Part model, mm, in its own coordinate system. Round coordinates to 2 decimals unless told otherwise and drop trailing zeros. Order: outer loops, then holes, each group sorted by start corner. A loop starts at its lowest first (then second) coordinate and runs counter-clockwise, first axis right, second up. Notation, with made-up numbers: (75, -18.5) - (90, -18.5) arc R16 cw to (90, 10.5) - close; hole circle Ø1 at (-7.75, -21). An arc over 180 degrees is marked (long way). Return JSON: item names as keys, results as strings. Group by question number.
Item 1: Two-plate mould, pull along X, no slides. Class faces 1 (the face through (80, 7, 1)), 2 (the face through (-1, 15, -1)), 3 (the face through (-12.39, 10.76, 20.32)), 4 (the face through (64.581, 5.196, -28.794)): released by +X, released by -X, zero draft, split by the parting line, or undercut.
Item 2: Saw through at B-B on z = -25. List the corners of the cut face in (x, y).
Item 3: Saw through at D-D on z = 0. List the corners of the cut face in (x, y), and give its area (3 significant figures).
Item 4: Saw through at C-C on y = 3. State how many separate pieces and enclosed holes the cut face has, and give its area (3 significant figures).
Item 5: Saw through at A-A on x = 0. List the corners of the cut face in (y, z), and give its area (4 significant figures).
Item 6: Probe probe 1 along Z at (x, y) = (-67, 4.5); probe 2 along X at (y, z) = (5, -33.75); probe 3 along Z at (x, y) = (14.5, 8.25). List the from-to ranges inside material, lowest first.
Item 7: Drop flat-ended pins along their axis: pin 1 (11.5 mm diameter, centred on x = -13, z = -25, fed in from +Y); pin 2 (14.5 mm diameter, centred on x = 13, z = 25, fed in from +Y). Give the stop position or say it passes through.
```python
from build123d import *

# Parameters (mm, degrees)
DODANIE_WYCI_GNI_CIE1_DEPTH                        = 15
SZKIC2_R                                           = 4
WYTNIJ_WYCI_GNI_CIE1_DEPTH                         = 103.621878759
LUSTRO2_COPY_1_SKETCH_R                            = 4
LUSTRO2_COPY_1_DEPTH                               = 103.621878759
SFAZOWANIE1_SIZE                                   = 0.5
POG_BIENIE_STO_KOWE_POD_M8_WKR_T_Z_BEM_D           = 9
POG_BIENIE_STO_KOWE_POD_M8_WKR_T_Z_BEM_CSINK_D     = 17.92
POG_BIENIE_STO_KOWE_POD_M8_WKR_T_Z_BEM_CSINK_ANGLE = 90
SZKIC5_R                                           = 4
WYTNIJ_WYCI_GNI_CIE2_DEPTH                         = 103.621878759


with BuildPart() as part:
    # Szkic1 → Dodanie-wyciągnięcie1 (new body)
    with BuildSketch(Plane(origin=(0, 0, 0), x_dir=(1, 0, 0), z_dir=(0, 1, 0))):
        with BuildLine():
            Line((-70, -62.5), (70, -62.5))
            ThreePointArc((70, -62.5), (77.071067812, -59.571067812), (80, -52.5))
            Line((80, -52.5), (80, 52.5))
            ThreePointArc((80, 52.5), (77.071067812, 59.571067812), (70, 62.5))
            Line((70, 62.5), (-70, 62.5))
            ThreePointArc((-70, 62.5), (-77.071067812, 59.571067812), (-80, 52.5))
            Line((-80, 52.5), (-80, -52.5))
            ThreePointArc((-80, -52.5), (-77.071067812, -59.571067812), (-70, -62.5))
        make_face()
    extrude(amount=DODANIE_WYCI_GNI_CIE1_DEPTH)

    # Szkic2 → Wytnij-wyciągnięcie1 (cut, symmetric)
    with BuildSketch(Plane(origin=(0, 15, 0), x_dir=(1, 0, 0), z_dir=(0, 1, 0))):
        with Locations(Location((-67, -25, 0), (0, 0, 270))):
            Circle(SZKIC2_R)
        with Locations(Location((-13, -25, 0), (0, 0, 90))):
            Circle(SZKIC2_R)
    wytnij_wyci_gni_cie1 = extrude(amount=WYTNIJ_WYCI_GNI_CIE1_DEPTH, both=True, mode=Mode.SUBTRACT)

    # Lustro1: Wytnij-wyciągnięcie1 across plane
    add(wytnij_wyci_gni_cie1.mirror(Plane.XY), mode=Mode.SUBTRACT)

    # Lustro2: Wytnij-wyciągnięcie1 across plane
    add(wytnij_wyci_gni_cie1.mirror(Plane(origin=(0, 0, 0), x_dir=(0, 0, 1), z_dir=(1, 0, 0))), mode=Mode.SUBTRACT)

    # Lustro2 copy 1 sketch → Lustro2 copy 1 (cut, symmetric)
    with BuildSketch(Plane(origin=(0, 15, 0), x_dir=(-1, 0, 0), z_dir=(0, 1, 0))):
        with Locations(Location((-67, -25, 0), (0, 0, 270))):
            Circle(LUSTRO2_COPY_1_SKETCH_R)
        with Locations(Location((-13, -25, 0), (0, 0, 90))):
            Circle(LUSTRO2_COPY_1_SKETCH_R)
    extrude(amount=LUSTRO2_COPY_1_DEPTH, both=True, mode=Mode.SUBTRACT)

    # Sfazowanie1
    sfazowanie1_edges = [part.edges().sort_by_distance(p)[0] for p in [
        (-67, 0, 21),
        (-67, 15, 21),
        (-13, 0, 29),
        (-13, 15, 29),
        (-67, 15, -21),
        (-67, 0, -21),
        (-13, 15, -29),
        (-13, 0, -29),
        (67, 0, -21),
        (67, 15, -21),
        (13, 0, -29),
        (13, 15, -29),
        (67, 15, 21),
        (67, 0, 21),
        (13, 15, 29),
        (13, 0, 29),
    ]]
    chamfer(sfazowanie1_edges, length=SFAZOWANIE1_SIZE)

    # Pogłębienie stożkowe pod M8 Wkręt z łbem stożkowym płaskim1 (through all)
    with Locations(Plane(origin=(0, 15, 0), x_dir=(1, 0, 0), z_dir=(0, 1, 0))):
        with Locations((-67, 25), (-13, 25), (-13, -25), (13, -25), (13, 25), (67, 25), (67, -25), (-67, -25)):
            CounterSinkHole(POG_BIENIE_STO_KOWE_POD_M8_WKR_T_Z_BEM_D / 2, POG_BIENIE_STO_KOWE_POD_M8_WKR_T_Z_BEM_CSINK_D / 2, counter_sink_angle=POG_BIENIE_STO_KOWE_POD_M8_WKR_T_Z_BEM_CSINK_ANGLE)

    # Szkic5 → Wytnij-wyciągnięcie2 (cut, through all)
    with BuildSketch(Plane(origin=(0, 15, 0), x_dir=(1, 0, 0), z_dir=(0, 1, 0))):
        with Locations(Location((0, 33.75, 0), (0, 0, 270))):
            Circle(SZKIC5_R)
        with Locations(Location((33.75, 0, 0), (0, 0, 270))):
            Circle(SZKIC5_R)
        with Locations(Location((0, -33.75, 0), (0, 0, 270))):
            Circle(SZKIC5_R)
        with Locations(Location((-33.75, 0, 0), (0, 0, 270))):
            Circle(SZKIC5_R)
    extrude(amount=-WYTNIJ_WYCI_GNI_CIE2_DEPTH, mode=Mode.SUBTRACT)


solid = part.part
```
Filled in:
{
 "1": {"face 1": "released by +X", "face 2": "zero draft", "face 3": "undercut", "face 4": "undercut"},
 "2": {"outline": "(-80, 0) - (-71.5, 0) - (-71.5, 10.54) - (-75.96, 15) - (-80, 15) - close; (-62.5, 0) - (-17.5, 0) - (-17.5, 10.54) - (-21.96, 15) - (-58.04, 15) - (-62.5, 10.54) - close; (-8.5, 0) - (8.5, 0) - (8.5, 10.54) - (4.04, 15) - (-4.04, 15) - (-8.5, 10.54) - close; (17.5, 0) - (62.5, 0) - (62.5, 10.54) - (58.04, 15) - (21.96, 15) - (17.5, 10.54) - close; (71.5, 0) - (80, 0) - (80, 15) - (75.96, 15) - (71.5, 10.54) - close"},
 "3": {"outline": "(-80, 0) - (-37.75, 0) - (-37.75, 15) - (-80, 15) - close; (-29.75, 0) - (29.75, 0) - (29.75, 15) - (-29.75, 15) - close; (37.75, 0) - (80, 0) - (80, 15) - (37.75, 15) - close", "area": "2,160 mm^2"},
 "4": {"separate pieces": "1", "enclosed holes": "12", "area": "19,200 mm^2"},
 "5": {"outline": "(0, -62.5) - (15, -62.5) - (15, -37.75) - (0, -37.75) - close; (0, -29.75) - (15, -29.75) - (15, 29.75) - (0, 29.75) - close; (0, 37.75) - (15, 37.75) - (15, 62.5) - (0, 62.5) - close", "area": "1,635 mm^2"},
 "6": {"probe 1": "z = -62.5 to -29.5, -20.5 to 20.5, 29.5 to 62.5", "probe 2": "x = -80 to -4, 4 to 80", "probe 3": "z = -62.5 to -29.24, -20.76 to 20.76, 29.24 to 62.5"},
 "7": {"pin 1": "stops at y = 11.79", "pin 2": "stops at y = 13.29"}
}
